Verification items for this drawing (mm, ordinates from the low corner). A direction names the side the tool comes from. Give positions to 0.01 mm unless a question says otherwise; leave off trailing zeros. Write each loop counter-clockwise with the first axis right and the second up, starting at its lowest first coordinate (ties: lowest second). Pieces come first, ordered by that corner, then holes. Notation, with made-up numbers: M 15.25,57 L 63.25,57 A18 ccw 63.25,83 Z; hole C 89,-13 d4. An arc over 180 degrees is marked long. Write each question's results on one line, items separated by ' | '.
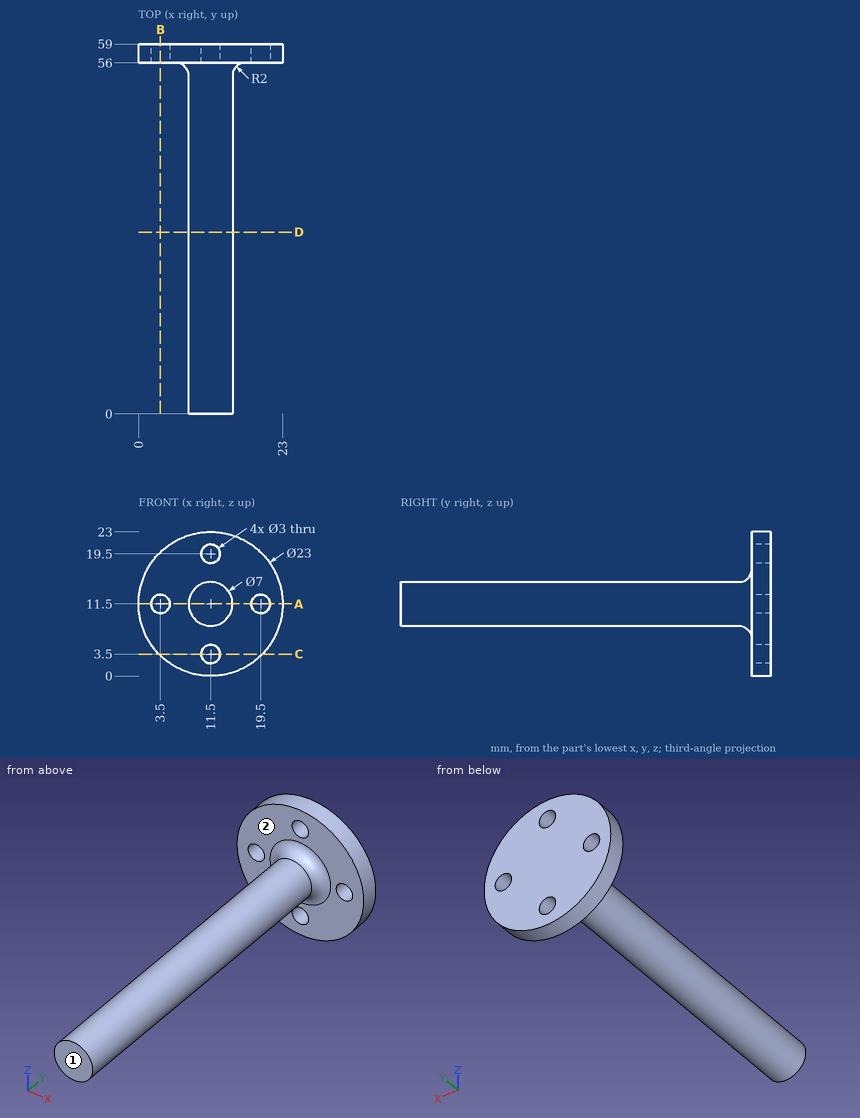
Q1. Depth check by flat-ended pin: P1, Ø3, axis at y = 31, z = 15.5, coming from the +X side; P2, Ø2.5, axis at x = 19.5, z = 11.5, coming from the +Y side; P3, Ø10, axis at x = 4.5, y = 34.5, coming from the +Z side; P4, Ø5, axis at x = 11.5, y = 47.5, coming from the +Z side. Enter the tip coordinate at first touch or a pass-through.
Answer key:
P1: stops at x = 13.95 | P2: passes through | P3: stops at z = 14.37 | P4: stops at z = 15
Q2. Material ranges on probe 1 along Z at (x, y) = (11.5, 57.9); probe 2 along Y at (x, z) = (8, 20.75); probe 3 along Z at (x, y) = (3.5, 56.7), recorded low to high. Write a range as [from, to].
Answer key:
probe 1: z = [0, 2], [5, 18], [21, 23] | probe 2: y = [56, 59] | probe 3: z = [3.24, 10], [13, 19.76]
Q3. Section check A-A (z = 11.5). Enter the section's corners in (x, y).
Answer key:
outline: M 0,56 L 2,56 L 2,59 L 0,59 Z; M 5,56 L 6,56 A2 cw 8,54 L 8,0 L 15,0 L 15,54 A2 cw 17,56 L 18,56 L 18,59 L 5,59 Z; M 21,56 L 23,56 L 23,59 L 21,59 Z
Q4. Access from +Z, -Z, +X, -X, +Y, -Y to the whole of each face (thin tool, end or side, straight path). Record for the marked faces 1 and 2.
Answer key:
face 1: +Z, -Z, +X, -X, -Y | face 2: -Y
Q5. Section check C-C (z = 3.5). Enter the section's corners in (x, y), then the cut area to 3 significant figures.
Answer key:
outline: M 3.24,56 L 10,56 L 10,59 L 3.24,59 Z; M 13,56 L 19.76,56 L 19.76,59 L 13,59 Z | area: 40.6 mm2
Q6. Section check B-B (x = 3.5). Enter the section's corners in (y, z), then the cut area to 3 significant figures.
Answer key:
outline: M 56,3.24 L 59,3.24 L 59,10 L 56,10 Z; M 56,13 L 59,13 L 59,19.76 L 56,19.76 Z | area: 40.6 mm2
Q7. Section check D-D (y = 29). Enter the section's corners in (x, z), then the cut area to 3 significant figures.
Answer key:
outline: C 11.5,11.5 d7 | area: 38.5 mm2
